from build123d import *

# Parameters (mm, degrees)
F1_DEPTH = 25.4
F2_R     = 2.15265
F3_DEPTH = 2.65684
F4_R     = 2.15265
F5_DEPTH = 2.65684
F6_R     = 3.08356
F7_R     = 5.7404


with BuildPart() as f1:
    # F0 (on Top) → F1 (new body)
    with BuildSketch(Plane.XY):
        Polygon((0, 2.65684), (0, 0), (48.14316, 0), (48.14316, -48.14316), (50.8, -48.14316), (50.8, 2.65684), align=None)
    extrude(amount=F1_DEPTH)

    # F2 (on face) → F3 (cut, through all)
    with BuildSketch(Plane(origin=(0, 2.65684, 0), x_dir=(-1, 0, 0), z_dir=(0, 1, 0))):
        with Locations((-12.7, 12.7)):
            Circle(F2_R)
    extrude(amount=-F3_DEPTH, mode=Mode.SUBTRACT)

    # F4 (on face) → F5 (cut, through all)
    with BuildSketch(Plane.YZ.offset(50.8)):
        with Locations((-22.74316, 12.7)):
            Circle(F4_R)
    extrude(amount=-F5_DEPTH, mode=Mode.SUBTRACT)

    # F6
    f6_edges = [f1.edges().sort_by_distance(p)[0] for p in [
        (48.14316, 0, 12.7),
    ]]
    fillet(f6_edges, radius=F6_R)

    # F7
    f7_edges = [f1.edges().sort_by_distance(p)[0] for p in [
        (50.8, 2.65684, 12.7),
    ]]
    fillet(f7_edges, radius=F7_R)


solid = f1.part
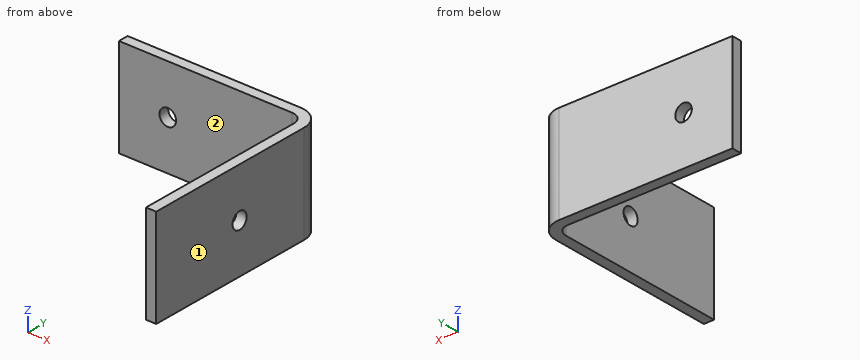
CAD build for the part. Positions are in the model's coordinates, mm. Face numbers are marked on the shaded views. A direction names the side the tool comes from. Coordinates: 2 decimals unless noted, no trailing zeros. Loops run counter-clockwise (first coordinate to the right, second up) from the corner with the lowest first, then second, coordinate; pieces in that order, holes last. Notation, with made-up numbers: (-39.75, 57) -> (15.25, 57) arc R19 ccw to (15.25, 82) -> close; hole circle Ø2 at (10.5, -31). An arc over 180 degrees is marked (long way). One line per item, written item: value.
1. Slice it at C-C on y = -23.5. Write the cut outline in (x, z).
Answers:
outline: (48.14, 0) -> (50.8, 0) -> (50.8, 10.68) -> (48.14, 10.68) -> close; (48.14, 14.72) -> (50.8, 14.72) -> (50.8, 25.4) -> (48.14, 25.4) -> close
2. Drill centre lines: line 1 (Z direction, x = 12.7, y = 1.05); line 2 (X direction, y = -6.5, z = 23); line 3 (Z direction, x = 12, y = 1). Where is each one in solid material? Low to high. Write a range as [from, to].
Answers:
line 1: z = [0, 10.55], [14.85, 25.4]
line 2: x = [48.14, 50.8]
line 3: z = [0, 10.66], [14.74, 25.4]
3. Slice it at B-B on z = 12.7. Write the cut outline in (x, y), and give its area (3 significant figures).
Answers:
outline: (0, 0) -> (10.55, 0) -> (10.55, 2.66) -> (0, 2.66) -> close; (14.85, 0) -> (45.06, 0) arc R3.08 cw to (48.14, -3.08) -> (48.14, -20.59) -> (50.8, -20.59) -> (50.8, -3.08) arc R5.74 ccw to (45.06, 2.66) -> (14.85, 2.66) -> close; (48.14, -48.14) -> (50.8, -48.14) -> (50.8, -24.9) -> (48.14, -24.9) -> close
area: 235 mm^2
4. Slice it at A-A on x = 12.7. Write the cut outline in (y, z), and give its area (3 significant figures).
Answers:
outline: (0, 0) -> (2.66, 0) -> (2.66, 10.55) -> (0, 10.55) -> close; (0, 14.85) -> (2.66, 14.85) -> (2.66, 25.4) -> (0, 25.4) -> close
area: 56.0 mm^2
5. Which spindle directions (+Z, -Z, +X, -X, +Y, -Y) get a long thin tool onto all of the face, cutting with end or side? Do the marked faces 1 and 2. Say none if no direction does.
Answers:
face 1: +Z, -Z, +X, +Y, -Y
face 2: +Z, -Z, -X, -Y
6. Slice it at D-D on z = 3.75. Write the cut outline in (x, y).
Answers:
outline: (0, 0) -> (45.06, 0) arc R3.08 cw to (48.14, -3.08) -> (48.14, -48.14) -> (50.8, -48.14) -> (50.8, -3.08) arc R5.74 ccw to (45.06, 2.66) -> (0, 2.66) -> close
7. Flat gauge pins, fed straight in: P1, Ø6, axis at x = 34.5, z = 10.5, coming from the -Y side; P2, Ø4, axis at x = 12.7, z = 12.7, coming from the -Y side; P3, Ø3, axis at y = -31, z = 10.5, coming from the -X side. Where does each tip first touch, or does it go through?
Answers:
P1: stops at y = 0
P2: passes through
P3: stops at x = 48.14
